Can you work these out from the drawing? Everything is in mm from the part's minimum corner. Round coordinates to 2 decimals unless told otherwise and drop trailing zeros. Write each loop counter-clockwise with the first axis right and the second up, starting at its lowest first coordinate (ties: lowest second). Pieces come first, ordered by that corner, then holes. Notation, with made-up numbers: (73, -14) - (98, -14) arc R21 cw to (98, 12) - close; hole circle Ø11 at (88, 39). An arc over 180 degrees is marked (long way). One line per item, written item: value. Start each with the question number.
Item 1: Imagine slicing it at A-A, the plane z = 3.5. Please give me the cut outline in (x, y), then the cut area to 3 significant figures.
Item 2: If I drill on line 1 (Y direction, x = 8.89, z = 1.5); line 2 (X direction, y = 5, z = 1) (1 decimal); line 3 (X direction, y = 45.5, z = 0.75) (1 decimal), over which ranges is the centre line in solid material (lowest first)?
Item 3: For P1, Ø1.9, axis at y = 73.5, z = 2.5, coming from the -X side; P2, Ø1, axis at y = 41.5, z = 2, coming from the +X side; P3, Ø1, axis at y = 9.5, z = 2, coming from the +X side, each with a flat end and sliding along its axis, tell me the tip position at first contact or that it passes through.
Item 4: Imagine slicing it at C-C, the plane y = 33. Please give me the cut outline in (x, z), then the cut area to 3 significant figures.
Item 5: Imagine slicing it at B-B, the plane x = 30. Please give me the cut outline in (y, z), then the cut area to 3 significant figures.
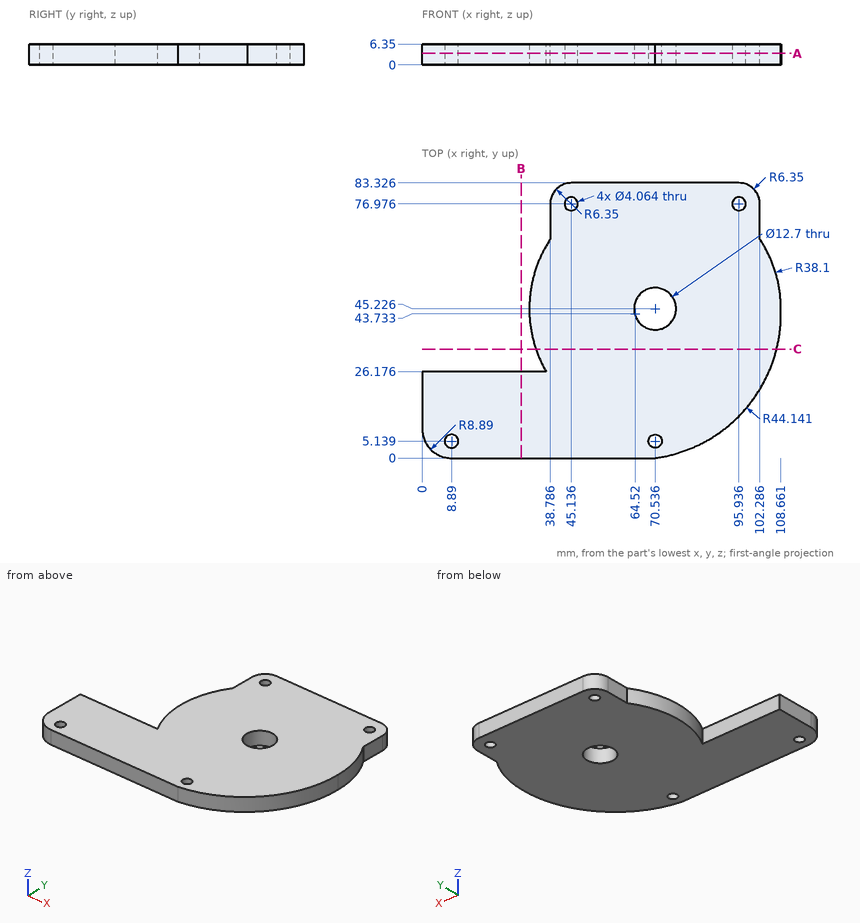
Values follow:
1. outline: (0, 8.89) arc R8.89 ccw to (8.89, 0) - (70.51, 0) arc R44.14 ccw to (108.64, 45.23) arc R38.1 ccw to (102.29, 66.29) - (102.29, 76.98) arc R6.35 ccw to (95.94, 83.33) - (45.14, 83.33) arc R6.35 ccw to (38.79, 76.98) - (38.79, 66.29) arc R38.1 ccw to (37.54, 26.18) - (0, 26.18) - close; hole circle Ø4.06 at (8.89, 5.14); hole circle Ø4.06 at (45.14, 76.98); hole circle Ø12.7 at (70.54, 45.23); hole circle Ø4.06 at (70.54, 5.14); hole circle Ø4.06 at (95.94, 76.98)
1. area: 6,250 mm^2
2. line 1: y = 0 to 3.11, 7.17 to 26.18
2. line 2: x = 0.9 to 6.9, 10.9 to 68.5, 72.6 to 85.7
2. line 3: x = 32.4 to 64.2, 76.9 to 108.6
3. P1: stops at x = 38.79
3. P2: stops at x = 108.63
3. P3: stops at x = 92.99
4. outline: (34.45, 0) - (107.34, 0) - (107.34, 6.35) - (34.45, 6.35) - close
4. area: 463 mm^2
5. outline: (0, 0) - (26.18, 0) - (26.18, 6.35) - (0, 6.35) - close
5. area: 166 mm^2
